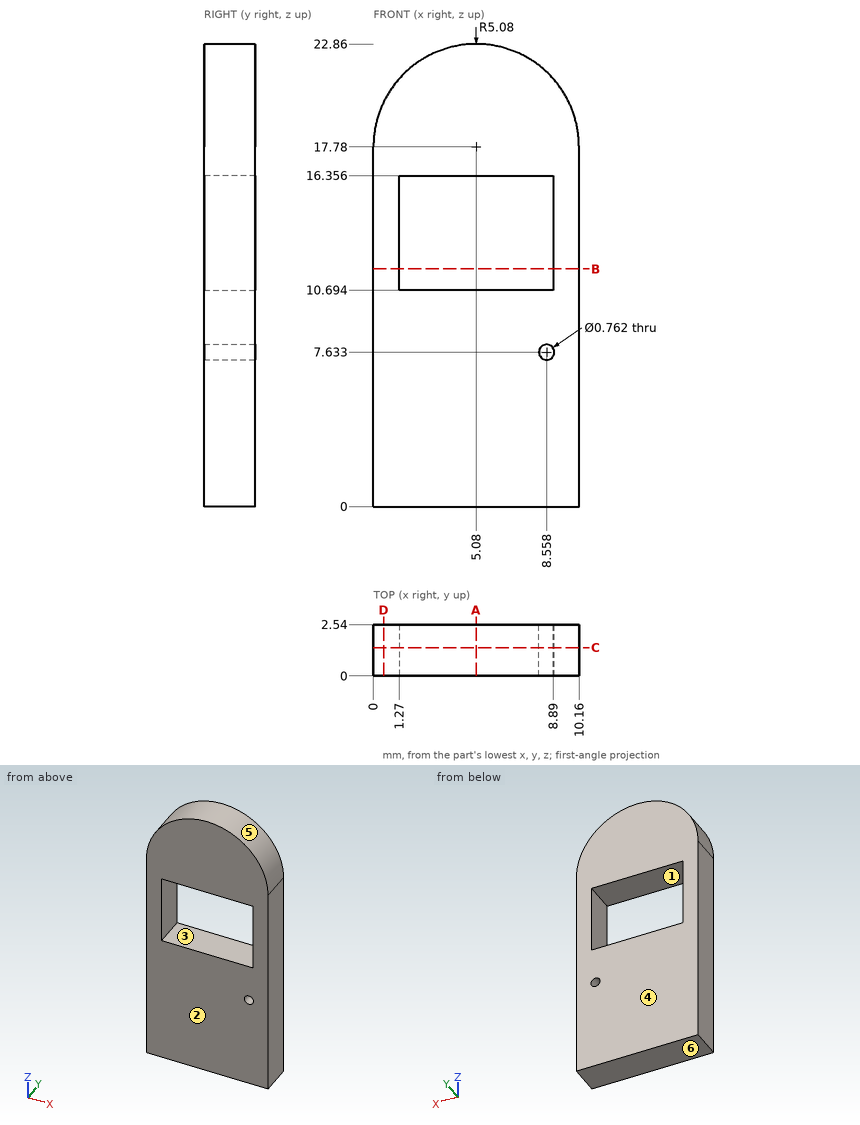
Design review of the part shown in the three views and the two pictorial views. Dimensions are in mm from the part's minimum x, y and z. A direction names the side the tool comes from. Give positions to 0.01 mm unless a question says otherwise; leave off trailing zeros. Write each loop counter-clockwise with the first axis right and the second up, starting at its lowest first coordinate (ties: lowest second). Pieces come first, ordered by that corner, then holes. Notation, with made-up numbers: M -3.5,-10.75 L 51.5,-10.75 A27 ccw 51.5,27.25 Z; hole C 67.5,-30.75 d5. An arc over 180 degrees is marked long. Return JSON: item names as keys, results as strings. Group by question number.
Item 1: The part is to be moulded in two halves that separate along Z. For the marked faces 3, 4, 5 and 6, say which applies: pulls with the +Z half, pulls with the -Z half, needs draft (parallel to the pull), parting line crosses it, or undercut.
Item 2: Take a section at A-A (x = 5.08). Give the boundary of the cut face in (y, z), plus the area to 3 significant figures.
Item 3: Wall thickness on line 1 along Z through (x, y) = (8.75, 2) (1 decimal); line 2 along X through (y, z) = (0.2, 12.25); line 3 along Z through (x, y) = (4, 1.3): over which ranges is each line inside the solid? List them lowest first.
Item 4: Take a section at C-C (y = 1.4). Give the boundary of the cut face in (x, z), plus the area to 3 significant figures.
Item 5: Tool access review of the marked faces 1 and 2: name each direction out of +Z, -Z, +X, -X, +Y, -Y from which nothing blocks a thin tool from reaching the whole face with its end or side.
Item 6: Clearance check with a flat-ended pin moving along its axis: pin 1 Ø0.8 at (x, y) = (4.5, 1.5) entering from +Z. State where the tip first meets the part, or that it passes through.
Item 7: Take a section at B-B (z = 11.75). Give the boundary of the cut face in (x, y).
Item 8: Take a section at D-D (x = 0.5). Give the boundary of the cut face in (y, z).
Return value:
{
 "1": {"face 3": "undercut", "face 4": "needs draft", "face 5": "pulls with the +Z half", "face 6": "pulls with the -Z half"},
 "2": {"outline": "M 0,0 L 2.54,0 L 2.54,10.69 L 0,10.69 Z; M 0,16.36 L 2.54,16.36 L 2.54,22.86 L 0,22.86 Z", "area": "43.7 mm2"},
 "3": {"line 1": "z = 0 to 7.3, 8 to 10.7, 16.4 to 21.3", "line 2": "x = 0 to 1.27, 8.89 to 10.16", "line 3": "z = 0 to 10.69, 16.36 to 22.74"},
 "4": {"outline": "M 0,0 L 10.16,0 L 10.16,17.78 A5.08 ccw 0,17.78 Z; hole M 1.27,10.69 L 8.89,10.69 L 8.89,16.36 L 1.27,16.36 Z; hole C 8.56,7.63 d0.76", "area": "178 mm2"},
 "5": {"face 1": "+Y, -Y", "face 2": "+Z, -Z, +X, -X, -Y"},
 "6": {"pin 1": "stops at z = 22.86"},
 "7": {"outline": "M 0,0 L 1.27,0 L 1.27,2.54 L 0,2.54 Z; M 8.89,0 L 10.16,0 L 10.16,2.54 L 8.89,2.54 Z"},
 "8": {"outline": "M 0,0 L 2.54,0 L 2.54,19.98 L 0,19.98 Z"}
}
